```python
from build123d import *

# Parameters (mm, degrees)
SKETCH_1_R      = 3
EXTRUDE_1_DEPTH = 3
SKETCH_2_R      = 0.293076877
EXTRUDE_2_DEPTH = 40
SCALE_1_SCALE   = 3.5


with BuildPart() as part:
    # 草图1 → 凸台-拉伸1 (new body)
    with BuildSketch(Plane.XY):
        with BuildLine():
            Line((8.2, 0.3), (3.189519169, 0.258780744))
            ThreePointArc((3.189519169, 0.258780744), (-3.199933121, 0.020688637), (3.185906464, -0.3))
            Line((3.185906464, -0.3), (8.2, -0.3))
            Line((8.2, -0.3), (8.2, 0.3))
        make_face()
        Circle(SKETCH_1_R, mode=Mode.SUBTRACT)
    extrude(amount=EXTRUDE_1_DEPTH)

    # 草图2 → 凸台-拉伸2 (add)
    with BuildSketch(Plane(origin=(8.2, 0, 0), x_dir=(0, 0, -1), z_dir=(1, 0, 0))):
        with Locations((-1.506058585, 0)):
            Circle(SKETCH_2_R)
    extrude(amount=EXTRUDE_2_DEPTH)


with BuildPart() as part_1:
    # 缩放比例1: scaled about (11.360396765, -0.00284627, 1.502097409)
    add(part.part.scale(SCALE_1_SCALE).moved(Location((-28.400991913, 0.007115675, -3.755243523))))


solid = part_1.part
```
Design review of the part built by this model. Coordinates are the model's own, in mm. A direction names the side the tool comes from. Coordinates: 2 decimals unless noted, no trailing zeros. Loops run counter-clockwise (first coordinate to the right, second up) from the corner with the lowest first, then second, coordinate; pieces in that order, holes last. Notation, with made-up numbers: (14.25, -14.75) -> (73.25, -14.75) arc R11 cw to (73.25, 1.25) -> close; hole circle Ø1 at (86.25, 57). An arc over 180 degrees is marked (long way). Answer as a JSON object with one key per item and string values.
Q1. Clearance check with flat-ended pins moving along their axes: pin 1 Ø4 at (y, z) = (-7.5, 3) entering from -X; pin 2 Ø1.7 at (y, z) = (-0.5, 3.5) entering from +X; pin 3 Ø2 at (x, z) = (120.5, 2) entering from -Y; pin 4 Ø2 at (x, z) = (59, 5) entering from +Y. State where each tip first meets the part, or that it passes through.
Answer block:
{"pin 1": "stops at x = -38.15", "pin 2": "stops at x = 0.3", "pin 3": "stops at y = -1.02", "pin 4": "passes through"}
Q2. Take a section at A-A on y = -5.25. Give the boundary of the cut face in (x, z), plus the area to 3 significant figures.
Answer block:
{"outline": "(-38.29, -3.76) -> (-37.49, -3.76) -> (-37.49, 6.74) -> (-38.29, 6.74) -> close; (-19.31, -3.76) -> (-18.51, -3.76) -> (-18.51, 6.74) -> (-19.31, 6.74) -> close", "area": "16.8 mm^2"}
Q3. Tool access review of faces 3 (the flat face through (-9, -1.043, 1)), 4 (the cylindrical face through (-39.587, 0.558, 1.421)): name each direction out of +Z, -Z, +X, -X, +Y, -Y from which nothing blocks a thin tool from reaching the whole face with its end or side.
Answer block:
{"face 3": "+Z, -Z, +X, -Y", "face 4": "+Z, -Z"}
Q4. Take a section at B-B on z = -1. Give the boundary of the cut face in (x, y), plus the area to 3 significant figures.
Answer block:
{"outline": "(-17.25, -1.04) -> (0.3, -1.04) -> (0.3, 1.06) -> (-17.24, 0.91) arc R11.2 ccw (long way) to start; hole circle Ø21 at (-28.4, 0.01)", "area": "83.2 mm^2"}
Q5. Take a section at C-C on x = -8.5. Give the boundary of the cut face in (y, z).
Answer block:
{"outline": "(-1.04, -3.76) -> (0.98, -3.76) -> (0.98, 6.74) -> (-1.04, 6.74) -> close"}
Q6. Take a section at D-D on y = 4. Give the boundary of the cut face in (x, z).
Answer block:
{"outline": "(-38.87, -3.76) -> (-38.11, -3.76) -> (-38.11, 6.74) -> (-38.87, 6.74) -> close; (-18.69, -3.76) -> (-17.94, -3.76) -> (-17.94, 6.74) -> (-18.69, 6.74) -> close"}
Q7. To check wall thickness, follow L1, parallel to Y at x = -2, z = 5.5; L2, parallel to X at y = -6.5, z = -0.25; L3, parallel to X at y = 6.25, z = 2.25. State the ranges of each line that lie inside material, in increasing order.
Answer block:
{"L1": "y = -1.04 to 1.04", "L2": "x = -37.52 to -36.64, -20.16 to -19.29", "L3": "x = -37.7 to -36.84, -19.96 to -19.1"}
Q8. The part is to be moulded in two halves that separate along X. For faces 1 (the cylindrical face through (-18.4, 3.2, 1.4)), 2 (the flat face through (-17, 0, -3.755)), say which applies: +X half, -X half, draft (parallel to the pull), parting line (faces both ways), or undercut.
Answer block:
{"face 1": "undercut", "face 2": "draft"}
